from build123d import *

# Parameters (mm, degrees)
CROQUIS1_W                 = 25
CROQUIS1_H                 = 25
CROQUIS1_R                 = 5.5
SALIENTE_EXTRUIR1_DEPTH    = 10
CORTAR_EXTRUIR1_REACH      = 38.742
CORTAR_EXTRUIR1_END_RADIUS = 5.5
CROQUIS2_R                 = 2
CROQUIS3_W                 = 3.068049468
CROQUIS3_H                 = 5.6
CORTAR_EXTRUIR2_DEPTH      = 37.742346169


with BuildPart() as part:
    # Croquis1 → Saliente-Extruir1 (new body)
    with BuildSketch(Plane.XY):
        with Locations((12.5, 12.5)):
            Rectangle(CROQUIS1_W, CROQUIS1_H)
        with Locations((12.5, 12.5)):
            Circle(CROQUIS1_R, mode=Mode.SUBTRACT)
    extrude(amount=SALIENTE_EXTRUIR1_DEPTH)

    # Cortar-Extruir1: up to this cylinder (the profile starts outside it)
    cortar_extruir1_end = Plane(origin=(12.5, 12.5, 4.2), z_dir=(0, 0, -1)) * Cylinder(CORTAR_EXTRUIR1_END_RADIUS, 89.484, mode=Mode.PRIVATE)
    # Croquis2 → Cortar-Extruir1 (cut, up to the surface)
    with BuildSketch(Plane.ZY, mode=Mode.PRIVATE) as cortar_extruir1_sk1:
        with Locations((4.2, 12.5)):
            Circle(CROQUIS2_R)
    cortar_extruir1_tool1 = extrude(cortar_extruir1_sk1.sketch, amount=-CORTAR_EXTRUIR1_REACH, mode=Mode.PRIVATE) - cortar_extruir1_end
    add(cortar_extruir1_tool1.solids().sort_by_distance((0, 12.5, 4.2))[0], mode=Mode.SUBTRACT)

    # Croquis3 → Cortar-Extruir2 (cut, through all)
    with BuildSketch(Plane(origin=(0, 0, 0), x_dir=(-1, 0, 0), z_dir=(0, 0, -1))):
        with Locations((-3.965975266, 12.5)):
            Rectangle(CROQUIS3_W, CROQUIS3_H)
    extrude(amount=-CORTAR_EXTRUIR2_DEPTH, mode=Mode.SUBTRACT)


solid = part.part
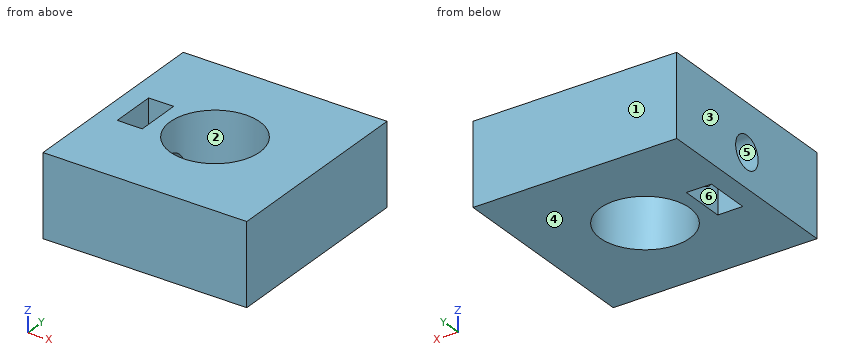
Could you check a few things on this model? Use its own coordinates, in mm. Face numbers are marked on the shaded views. A direction names the side the tool comes from. Give positions to 0.01 mm unless a question says otherwise; leave off trailing zeros. Write each loop counter-clockwise with the first axis right and the second up, starting at its lowest first coordinate (ties: lowest second). Pieces come first, ordered by that corner, then holes. Notation, with made-up numbers: (-0.75, -25) -> (55.25, -25) arc R7 ccw to (55.25, -20) -> close; hole circle Ø4 at (-26.75, -14.75). An arc over 180 degrees is marked (long way). Answer as a JSON object with one key per item and string values.
Q1. Please list where these lines run through material, in increasing order: L1, parallel to Y at x = 6.6, z = 4.2; L2, parallel to Z at x = 6.55, y = 12.5; L3, parallel to Y at x = 2.5, z = 9.
Taken from the geometry:
{"L1": "y = 0 to 10.5, 14.5 to 25", "L2": "z = 0 to 2.2, 6.2 to 10", "L3": "y = 0 to 9.7, 15.3 to 25"}
Q2. Suppose I cut it at B-B on z = 6.75. Write out the boundary of the cut face in (x, y), then the cut area to 3 significant figures.
Taken from the geometry:
{"outline": "(0, 0) -> (25, 0) -> (25, 25) -> (0, 25) -> close; hole (2.43, 9.7) -> (5.5, 9.7) -> (5.5, 15.3) -> (2.43, 15.3) -> close; hole circle Ø11 at (12.5, 12.5)", "area": "513 mm²"}
Q3. Suppose I cut it at C-C on y = 12.5. Write out the boundary of the cut face in (x, z), then the cut area to 3 significant figures.
Taken from the geometry:
{"outline": "(0, 0) -> (2.43, 0) -> (2.43, 2.2) -> (0, 2.2) -> close; (0, 6.2) -> (2.43, 6.2) -> (2.43, 10) -> (0, 10) -> close; (5.5, 0) -> (7, 0) -> (7, 2.2) -> (5.5, 2.2) -> close; (5.5, 6.2) -> (7, 6.2) -> (7, 10) -> (5.5, 10) -> close; (18, 0) -> (25, 0) -> (25, 10) -> (18, 10) -> close", "area": "93.6 mm²"}
Q4. Suppose I cut it at A-A on x = 4.75. Write out the boundary of the cut face in (y, z), then the cut area to 3 significant figures.
Taken from the geometry:
{"outline": "(0, 0) -> (9.7, 0) -> (9.7, 10) -> (0, 10) -> close; (15.3, 0) -> (25, 0) -> (25, 10) -> (15.3, 10) -> close", "area": "194 mm²"}
Q5. We'd pull the mould along X, two halves only. Please class the marked faces 1, 2 and 3: released by +X, released by -X, zero draft, split by the parting line, or undercut.
Taken from the geometry:
{"face 1": "zero draft", "face 2": "undercut", "face 3": "released by -X"}
Q6. Which directions (+Z, -Z, +X, -X, +Y, -Y) give clear straight access to the entire face, cutting with the end or side of a thin tool? Please do the marked faces 4, 5 and 6.
Taken from the geometry:
{"face 4": "-Z, +X, -X, +Y, -Y", "face 5": "-X", "face 6": "+Z, -Z"}
Q7. Suppose I cut it at D-D on x = 12.5. Write out the boundary of the cut face in (y, z), then the cut area to 3 significant figures.
Taken from the geometry:
{"outline": "(0, 0) -> (7, 0) -> (7, 10) -> (0, 10) -> close; (18, 0) -> (25, 0) -> (25, 10) -> (18, 10) -> close", "area": "140 mm²"}
